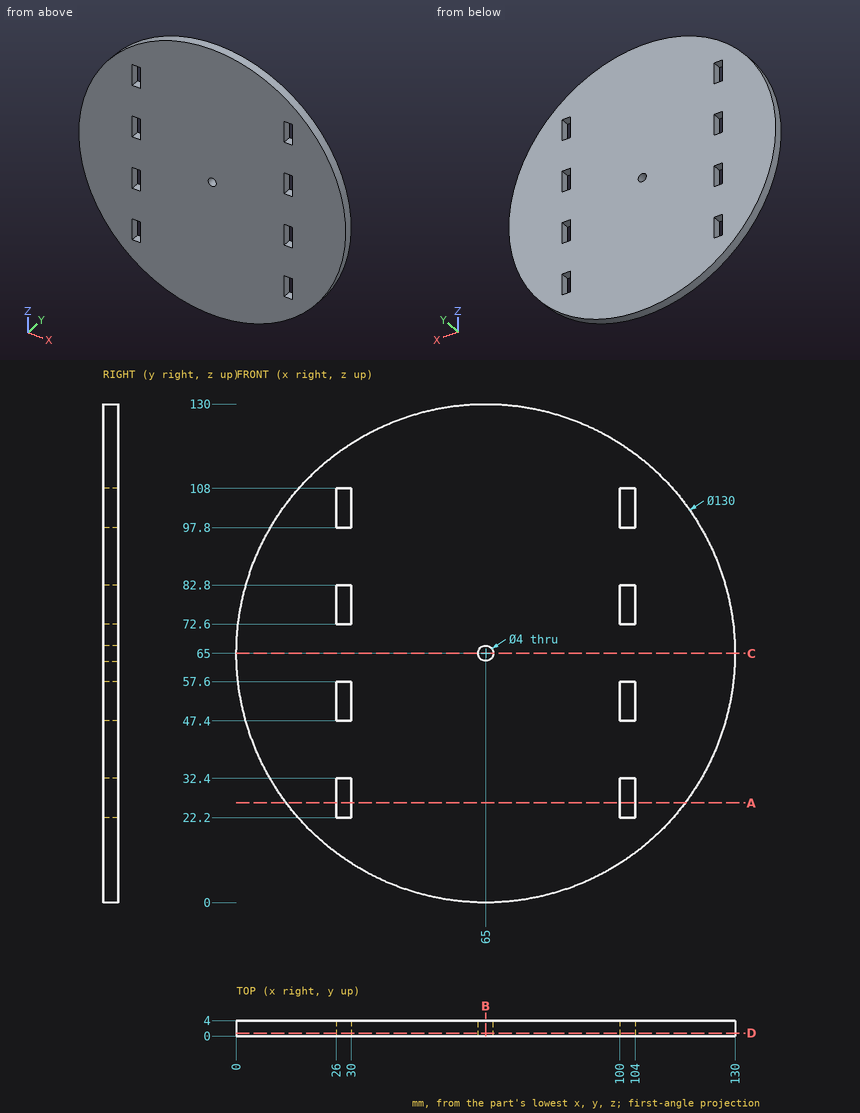
The drawing under review shows one solid part. Ordinate dimensions are in mm from its lowest x, y, z. Coordinates: 2 decimals unless noted, no trailing zeros. Write each loop counter-clockwise with the first axis right and the second up, starting at its lowest first coordinate (ties: lowest second). Pieces come first, ordered by that corner, then holes. Notation, with made-up numbers: (-31.75, 54.5) - (1.25, 54.5) arc R29 cw to (1.25, 84.5) - close; hole circle Ø9 at (-21, 54). An arc over 180 degrees is marked (long way). Put each result on its own line as item: value.
1. Wall thickness on probe 1 along X at (y, z) = (1.7, 65); probe 2 along X at (y, z) = (2, 77); probe 3 along X at (y, z) = (2.55, 52): over which ranges is each line inside the solid? List them lowest first.
Values found:
probe 1: 0 to 63, 67 to 130
probe 2: 1.12 to 26, 30 to 100, 104 to 128.88
probe 3: 1.31 to 26, 30 to 100, 104 to 128.69
2. For pin 1 (2 mm diameter, centred on x = 102, y = 2.5, fed in from -Z); pin 2 (1.2 mm diameter, centred on y = 2.5, z = 26, fed in from +X); pin 3 (2 mm diameter, centred on y = 1.5, z = 27.5, fed in from -X); pin 4 (3 mm diameter, centred on x = 28.5, z = 86.5, fed in from -Y), all flat-tipped, find the tip position at first contact; note any pin that passes through.
Values found:
pin 1: z = 10.88
pin 2: x = 117.44
pin 3: x = 11.22
pin 4: y = 0
3. Add section A-A, the plane z = 26. Give the boundary of the cut face in (x, y), then the cut area to 3 significant figures.
Values found:
outline: (13, 0) - (26, 0) - (26, 4) - (13, 4) - close; (30, 0) - (100, 0) - (100, 4) - (30, 4) - close; (104, 0) - (117, 0) - (117, 4) - (104, 4) - close
area: 384 mm²
4. Add section C-C, the plane z = 65. Give the boundary of the cut face in (x, y).
Values found:
outline: (0, 0) - (63, 0) - (63, 4) - (0, 4) - close; (67, 0) - (130, 0) - (130, 4) - (67, 4) - close
5. Add section D-D, the plane y = 0.75. Count the separate pieces of the cut face and the enclosed holes in it, then the cut area to 3 significant figures.
Values found:
separate pieces: 1
enclosed holes: 9
area: 12,900 mm²
6. Add section B-B, the plane x = 65. Give the boundary of the cut face in (y, z), then the cut area to 3 significant figures.
Values found:
outline: (0, 0) - (4, 0) - (4, 63) - (0, 63) - close; (0, 67) - (4, 67) - (4, 130) - (0, 130) - close
area: 504 mm²
